Can you work these out from the model? Positions are in its coordinate system, mm. Face numbers are marked on the shaded views. Give positions to 0.01 mm unless a question says otherwise; leave off trailing zeros. Write each loop counter-clockwise with the first axis right and the second up, starting at its lowest first coordinate (ties: lowest second). Pieces come first, ordered by that corner, then holes. Notation, with made-up numbers: (-26.5, 20) -> (27.5, 20) arc R6 ccw to (27.5, 28) -> close; hole circle Ø2 at (-28, 85.25). An arc over 180 degrees is marked (long way). Answer as CSV lines item,"result". Start each with the question number.
1. If we section it at A-A on z = 0: Write out the boundary of the cut face in (x, y), plus the area to 3 significant figures.
2. I need wall thicknesses on line 1 (X direction, y = -0.3, z = 0); line 2 (Y direction, x = 20.5, z = 2); line 3 (X direction, y = 0.4, z = 0). Which ranges of each line are inside material? Lowest first, please. Write a range as [from, to].
3. I'm going to push a flat-ended pin straight in: P1, Ø19, axis at x = 0, z = 0, coming from the -Y side. Where does the tip first touch, or does it pass through?
4. If we section it at C-C on y = 1.45: Write out the boundary of the cut face in (x, z).
5. If we mould it in two halves opening along X, with no side actions, what happens to the marked faces 1 and 2? For each: pulls with the +X half, pulls with the -X half, needs draft (parallel to the pull), parting line crosses it, or undercut.
6. If we section it at B-B on x = 0: Write out the boundary of the cut face in (y, z).
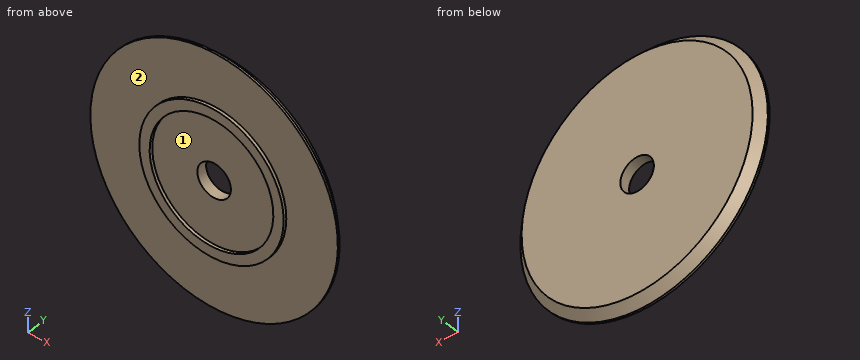
```python
from build123d import *

# Parameters (mm, degrees)
SKIZZE1_R                       = 24
SKIZZE1_R_2                     = 3.25
AUFSATZ_LINEAR_AUSTRAGEN1_DEPTH = 2
FASE1_SIZE                      = 1.6
SKIZZE2_R                       = 14
SKIZZE2_R_2                     = 12
AUFSATZ_LINEAR_AUSTRAGEN2_DEPTH = 0.6


with BuildPart() as part:
    # Skizze1 → Aufsatz-Linear austragen1 (new body)
    with BuildSketch(Plane(origin=(0, 0, 0), x_dir=(1, 0, 0), z_dir=(0, 1, 0))):
        with Locations(Location((0, 0, 0), (0, 0, 270))):
            Circle(SKIZZE1_R)
        with Locations(Location((0, 0, 0), (0, 0, 270))):
            Circle(SKIZZE1_R_2, mode=Mode.SUBTRACT)
    extrude(amount=AUFSATZ_LINEAR_AUSTRAGEN1_DEPTH)

    # Fase1
    fase1_edges = [part.edges().sort_by_distance(p)[0] for p in [
        (0, 2, -24),
    ]]
    chamfer(fase1_edges, length=FASE1_SIZE)

    # Skizze2 → Aufsatz-Linear austragen2 (add)
    with BuildSketch(Plane.XZ):
        with Locations(Location((0, 0, 0), (0, 0, 90))):
            Circle(SKIZZE2_R)
        with Locations(Location((0, 0, 0), (0, 0, 270))):
            Circle(SKIZZE2_R_2, mode=Mode.SUBTRACT)
    extrude(amount=AUFSATZ_LINEAR_AUSTRAGEN2_DEPTH)


solid = part.part
```
Computed values:
1,outline,"(-24, 0) -> (-14, 0) -> (-14, -0.6) -> (-12, -0.6) -> (-12, 0) -> (-3.25, 0) -> (-3.25, 2) -> (-22.4, 2) -> (-24, 0.4) -> close; (3.25, 0) -> (12, 0) -> (12, -0.6) -> (14, -0.6) -> (14, 0) -> (24, 0) -> (24, 0.4) -> (22.4, 2) -> (3.25, 2) -> close"
1,area,"82.8 mm2"
2,line 1,"x = [-14, -12], [12, 14]"
2,line 2,"y = [0, 2]"
2,line 3,"x = [-24, -3.25], [3.25, 24]"
3,P1,"stops at y = 0"
4,outline,"circle Ø45.9 at (0, 0); hole circle Ø6.5 at (0, 0)"
5,face 1,"undercut"
5,face 2,"needs draft"
6,outline,"(-0.6, -14) -> (0, -14) -> (0, -24) -> (0.4, -24) -> (2, -22.4) -> (2, -3.25) -> (0, -3.25) -> (0, -12) -> (-0.6, -12) -> close; (-0.6, 12) -> (0, 12) -> (0, 3.25) -> (2, 3.25) -> (2, 22.4) -> (0.4, 24) -> (0, 24) -> (0, 14) -> (-0.6, 14) -> close"
